Autodesk Inventor part; units mm, degrees
ref_plane "YZ Plane" through (0, 0, 0) normal (1, 0, 0) x (0, 1, 0)
ref_plane "XZ Plane" through (0, 0, 0) normal (0, 1, 0) x (-1, 0, 0)
ref_plane "XY Plane" through (0, 0, 0) normal (0, 0, 1) x (1, 0, 0)
sketch "스케치1" plane through (0, 0, 0) normal (0, 1, 0) x (-1, 0, 0)
  line L0 (-60, 100) -> (60, 100)
  line L1 (60, 100) -> (60, -100)
  line L2 (60, -100) -> (-60, -100)
  line L3 (-60, -100) -> (-60, 100)
  line L4 (-60, 100) -> (60, -100) construction
  line L5 (60, 100) -> (-60, -100) construction
  point P0 (0, 0)
  dimension "d0" = 200
  dimension "d1" = 120
extrude "돌출1" add sketch "스케치1" along normal blind 3
sketch "스케치2" plane through (0, 3, 0) normal (0, 1, 0) x (1, 0, 0)
  circle A0 centre (-15, -1) radius 10
  line L0 (-60, 100) -> (-60, -100)
  line L1 (60, 100) -> (-60, 100)
  point P0 (0, 0)
  dimension "d4" = 20
  dimension "d5" = 45
  dimension "d6" = 101
extrude "돌출2" cut sketch "스케치2" against normal through all
sketch "스케치3" plane through (0, 3, 0) normal (0, 1, 0) x (1, 0, 0)
  line L0 (-60, 25) -> (-57, 25)
  line L1 (-57, 25) -> (-57, 100)
  line L2 (-57, 100) -> (-60, 100)
  line L3 (-60, 100) -> (-60, 25)
  line L4 (-60, 100) -> (-60, -100)
  line L5 (60, 100) -> (-60, 100)
  line L6 (-60, 100) -> (-60, -100)
  line L7 (-60, 0) -> (60, 0)
  line L8 (60, -100) -> (60, 100)
  line L9 (60, 100) -> (-60, 100)
  line L10 (0, 100) -> (0, -100)
  line L11 (-60, -100) -> (60, -100)
  line L12 (-60, -25) -> (-57, -25)
  line L13 (-57, -25) -> (-57, -100)
  line L14 (-57, -100) -> (-60, -100)
  line L15 (-60, -100) -> (-60, -25)
  line L16 (60, 25) -> (57, 25)
  line L17 (57, 25) -> (57, 100)
  line L18 (57, 100) -> (60, 100)
  line L19 (60, 100) -> (60, 25)
  line L20 (60, 100) -> (60, -100)
  line L21 (60, 100) -> (60, -100)
  line L22 (60, -25) -> (57, -25)
  line L23 (57, -25) -> (57, -100)
  line L24 (57, -100) -> (60, -100)
  line L25 (60, -100) -> (60, -25)
  point P0 (0, 0)
  point P1 (-60, -100)
  point P2 (60, -100)
  point P3 (60, 25)
  point P4 (60, -25)
  point P5 (-60, -25)
  dimension "d9" = 75
  dimension "d10" = 3
extrude "돌출3" cut sketch "스케치3" against normal through all contours L3 L2 L1 L0 | L12 L13 L11 L4 | L5 L8 L16 L17 | L8 L11 L23 L22
sketch "스케치4" plane through (0, 3, 0) normal (0, 1, 0) x (1, 0, 0)
  line L0 (-57, -100) -> (57, -100)
  line L1 (57, -100) -> (15, -100)
  line L2 (15, -100) -> (15, -97)
  line L3 (15, -97) -> (57, -97)
  line L4 (57, -97) -> (57, -100)
  line L5 (0, -100) -> (0, 100)
  line L6 (57, 100) -> (-57, 100)
  line L7 (-59.774, 0) -> (60, 0)
  line L8 (60, -25) -> (60, 25)
  line L9 (57, 100) -> (15, 100)
  line L10 (15, 100) -> (15, 97)
  line L11 (15, 97) -> (57, 97)
  line L12 (57, 97) -> (57, 100)
  line L13 (-57, -100) -> (-15, -100)
  line L14 (-15, -100) -> (-15, -97)
  line L15 (-15, -97) -> (-57, -97)
  line L16 (-57, -97) -> (-57, -100)
  line L17 (-57, 100) -> (-15, 100)
  line L18 (-15, 100) -> (-15, 97)
  line L19 (-15, 97) -> (-57, 97)
  line L20 (-57, 97) -> (-57, 100)
  point P0 (0, 0)
  point P1 (-15, 100)
  point P2 (15, 100)
  point P3 (-15, -100)
  dimension "d13" = 3
  dimension "d14" = 42
extrude "돌출4" cut sketch "스케치4" against normal through all
sketch "스케치5" plane through (0, 3, 0) normal (0, 1, 0) x (1, 0, 0)
  point P0 (0, 0)
sketch "스케치6" plane through (0, 3, 0) normal (0, 1, 0) x (1, 0, 0)
  point P0 (0, 0)
properties part number "본체 뚜껑 레이저 수정"
Design review of the part built by this model. Coordinates are the model's own, in mm. Coordinates: 2 decimals unless noted, no trailing zeros. Order: outer loops, then holes, each group sorted by start corner. A loop starts at its lowest first (then second) coordinate and runs counter-clockwise, first axis right, second up. Notation, with made-up numbers: (44.25, 22) -> (94.25, 22) arc R32 cw to (94.25, 60) -> close; hole circle Ø9 at (84, 86.25). An arc over 180 degrees is marked (long way). One line per item, written item: value. Start each with the question number.
Q1. Take a section at C-C, the plane x = 24. State the section outline as (y, z) points, then the cut area to 3 significant figures.
Q2. Take a section at A-A, the plane z = 1. State the section outline as (x, y) points, then the cut area to 3 significant figures.
Q3. Insertion check: pin 1 Ø1.5 at (x, y) = (59, 1.5) entering from -Z; pin 2 Ø0.9 at (y, z) = (1.5, 98.5) entering from -X; pin 3 Ø12 at (x, z) = (-15, 1) entering from +Y; pin 4 Ø1.5 at (y, z) = (1, 57.5) entering from +X. Each pin has a flat end and moves straight along its axis. Give the tip position at first contact, or say it passes through.
Q4. Take a section at B-B, the plane y = 2.55. State the section outline as (x, z) points, then the cut area to 3 significant figures.
Q5. Mouldability with a two-part tool opening along Z and no side actions: class faces 1 (the flat face through (1, 0, 1)), 2 (the cylindrical face through (-5.763, 1.521, 4.83)) as pulls with the +Z half, pulls with the -Z half, needs draft (parallel to the pull), parting line crosses it, or undercut.
Q6. For probe 1 along X at (y, z) = (1.95, 1); probe 2 along X at (y, z) = (1.6, -54); probe 3 along Z at (x, y) = (-44.5, 1.9), list the stretches that pass through material, from the lowest coordinate up.
Q7. Take a section at D-D, the plane z = 72. State the section outline as (x, y) points, then the cut area to 3 significant figures.
Values follow:
1. outline: (0, -97) -> (3, -97) -> (3, 97) -> (0, 97) -> close
1. area: 582 mm2
2. outline: (-60, 0) -> (-25, 0) -> (-25, 3) -> (-60, 3) -> close; (-5, 0) -> (60, 0) -> (60, 3) -> (-5, 3) -> close
2. area: 300 mm2
3. pin 1: stops at z = -25
3. pin 2: stops at x = -15
3. pin 3: passes through
3. pin 4: stops at x = 57
4. outline: (-60, -25) -> (-57, -25) -> (-57, -97) -> (-15, -97) -> (-15, -100) -> (15, -100) -> (15, -97) -> (57, -97) -> (57, -25) -> (60, -25) -> (60, 25) -> (57, 25) -> (57, 97) -> (15, 97) -> (15, 100) -> (-15, 100) -> (-15, 97) -> (-57, 97) -> (-57, 25) -> (-60, 25) -> close; hole circle Ø20 at (-15, 1)
4. area: 22,300 mm2
5. face 1: needs draft
5. face 2: undercut
6. probe 1: x = -60 to -25, -5 to 60
6. probe 2: x = -57 to 57
6. probe 3: z = -97 to 97
7. outline: (-57, 0) -> (57, 0) -> (57, 3) -> (-57, 3) -> close
7. area: 342 mm2
